Source: three-view drawing plus pictorial views. Frame: mm from the lowest corner of the part. Give positions to 0.01 mm unless a question says otherwise; leave off trailing zeros. Order: outer loops, then holes, each group sorted by start corner. A loop starts at its lowest first (then second) coordinate and runs counter-clockwise, first axis right, second up. Notation, with made-up numbers: (62, 41.5) - (100, 41.5) arc R32 ccw to (100, 76.5) - close; hole circle Ø2 at (69, 55). An arc over 180 degrees is marked (long way). Use one line per item in the form item = value.
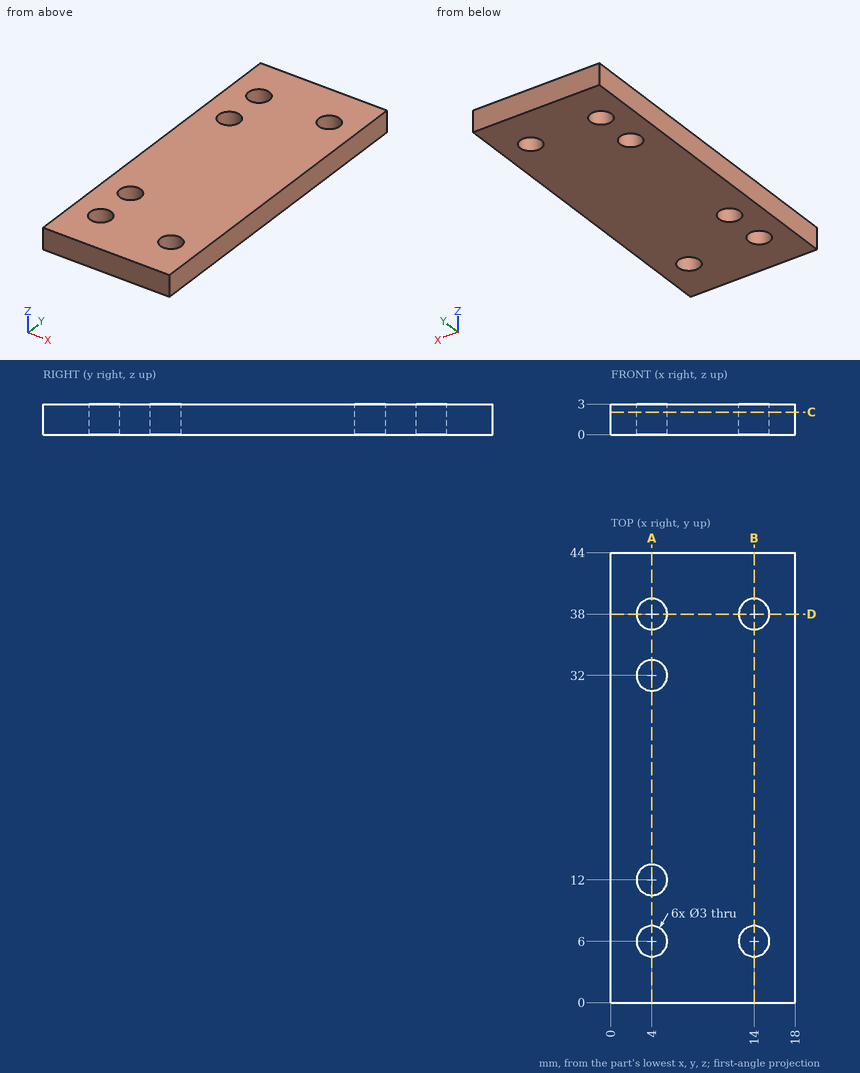
(1) Ray query, line 1 along X through (y, z) = (38, 0.7); line 2 along Y through (x, z) = (14, 0.75); line 3 along Y through (x, z) = (4, 0.8). Return the intervals inside material, ascending.
Computed values:
line_1 = 0 to 2.5, 5.5 to 12.5, 15.5 to 18
line_2 = 0 to 4.5, 7.5 to 36.5, 39.5 to 44
line_3 = 0 to 4.5, 7.5 to 10.5, 13.5 to 30.5, 33.5 to 36.5, 39.5 to 44
(2) Cut plane B-B on x = 14. Output: boundary loops of the cut face in (y, z).
Computed values:
outline = (0, 0) - (4.5, 0) - (4.5, 3) - (0, 3) - close; (7.5, 0) - (36.5, 0) - (36.5, 3) - (7.5, 3) - close; (39.5, 0) - (44, 0) - (44, 3) - (39.5, 3) - close
(3) Contact query for flat-ended pins moving along their axis: pin 1 Ø2.5 at (x, y) = (14, 38) entering from -Z; pin 2 Ø3.5 at (x, y) = (4, 38) entering from -Z. Output: stop coordinate, or through.
Computed values:
pin_1 = through
pin_2 = 0
(4) Cut plane D-D on y = 38. Output: boundary loops of the cut face in (x, z), plus the area to 3 significant figures.
Computed values:
outline = (0, 0) - (2.5, 0) - (2.5, 3) - (0, 3) - close; (5.5, 0) - (12.5, 0) - (12.5, 3) - (5.5, 3) - close; (15.5, 0) - (18, 0) - (18, 3) - (15.5, 3) - close
area = 36.0 mm²
(5) Cut plane A-A on x = 4. Output: boundary loops of the cut face in (y, z).
Computed values:
outline = (0, 0) - (4.5, 0) - (4.5, 3) - (0, 3) - close; (7.5, 0) - (10.5, 0) - (10.5, 3) - (7.5, 3) - close; (13.5, 0) - (30.5, 0) - (30.5, 3) - (13.5, 3) - close; (33.5, 0) - (36.5, 0) - (36.5, 3) - (33.5, 3) - close; (39.5, 0) - (44, 0) - (44, 3) - (39.5, 3) - close
(6) Cut plane C-C on z = 2.2. Output: boundary loops of the cut face in (x, y), plus the area to 3 significant figures.
Computed values:
outline = (0, 0) - (18, 0) - (18, 44) - (0, 44) - close; hole circle Ø3 at (4, 6); hole circle Ø3 at (4, 12); hole circle Ø3 at (4, 32); hole circle Ø3 at (4, 38); hole circle Ø3 at (14, 6); hole circle Ø3 at (14, 38)
area = 750 mm²
